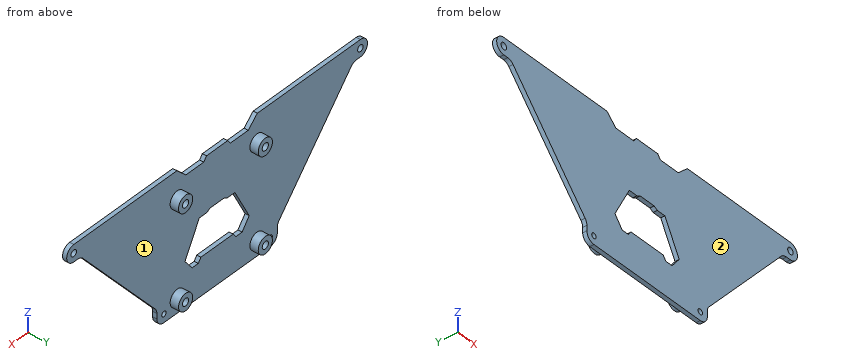
Autodesk Inventor part; units mm, degrees
ref_plane "YZ Plane" through (0, 0, 0) normal (1, 0, 0) x (0, 1, 0)
ref_plane "XZ Plane" through (0, 0, 0) normal (0, 1, 0) x (-1, 0, 0)
ref_plane "XY Plane" through (0, 0, 0) normal (0, 0, 1) x (1, 0, 0)
sketch "Sketch1" plane through (0, 0, 0) normal (0, 1, 0) x (-1, 0, 0)
  circle A0 centre (-13, 3.6355) radius 1.25
  circle A1 centre (47, 3.6355) radius 1.25
  circle A2 centre (-63.9, 60.95) radius 1.55
  circle A3 centre (-63.9, 60.95) radius 1.5
  circle A4 centre (97.9, 60.95) radius 1.55
  circle A5 centre (97.9, 60.95) radius 1.5
  arc A6 (47, -0.3645) -> (51, 3.6355) centre (47, 3.6355) ccw
  arc A7 (-17, 3.6355) -> (-13, -0.3645) centre (-13, 3.6355) ccw
  arc A8 (-63.9, 64.95) -> (-63.9, 56.95) centre (-63.9, 60.95) ccw
  arc A9 (97.9, 56.95) -> (97.9, 64.95) centre (97.9, 60.95) ccw
  line L0 (-13, -0.3645) -> (47, -0.3645)
  line L1 (-63.9, 64.95) -> (97.9, 64.95)
  line L2 (-17, 3.6355) -> (-17, 6.1391)
  line L3 (51, 3.6355) -> (51, 6.1391)
  arc A10 (51, 3.6355) -> (47, -0.3645) centre (47, 3.6355) ccw construction
  arc A11 (-13, -0.3645) -> (-17, 3.6355) centre (-13, 3.6355) ccw construction
  line L4 (-63.9, 56.95) -> (-61.722, 56.95)
  line L5 (97.9, 56.95) -> (95.722, 56.95)
  line L6 (92.7041, 55.5753) -> (51.9821, 8.7645)
  line L7 (-58.7041, 55.5753) -> (-17.9821, 8.7645)
  arc A12 (-58.7041, 55.5753) -> (-61.722, 56.95) centre (-61.722, 52.95) ccw
  arc A13 (95.722, 56.95) -> (92.7041, 55.5753) centre (95.722, 52.95) ccw
  arc A14 (51.9821, 8.7645) -> (51, 6.1391) centre (55, 6.1391) ccw
  arc A15 (-17, 6.1391) -> (-17.9821, 8.7645) centre (-21, 6.1391) ccw
  arc A16 (-63.9, 56.95) -> (-63.9, 64.95) centre (-63.9, 60.95) ccw construction
  arc A17 (97.9, 64.95) -> (97.9, 56.95) centre (97.9, 60.95) ccw construction
  point P0 (0, 0)
  point P1 (17, 90.5)
  dimension "d0" = 2.5
  dimension "d1" = 2.5
  dimension "d2" = 3
  dimension "d3" = 3
  dimension "d4" = 8
  dimension "d5" = 8
  dimension "d6" = 8
  dimension "d7" = 8
  dimension "d8" = 60
  dimension "d18" = 4
extrude "Extrusion1" add sketch "Sketch1" along normal blind 2 contours L0 A7 L2 A15 L7 A12 L4 A8 L1 A9 L5 A13 L6 A14 L3 A6
sketch "Sketch2" plane through (0, 2, 0) normal (0, 1, 0) x (1, 0, 0)
  circle A0 centre (13, -3.6355) radius 1.25
  circle A1 centre (-47, -3.6355) radius 1.25
  circle A2 centre (-39.5, -6.6355) radius 4
  circle A3 centre (5.5, -6.6355) radius 4
  circle A4 centre (5.5, -51.6355) radius 4
  circle A5 centre (-39.5, -51.6355) radius 4
  line L0 (13, 0.3645) -> (-47, 0.3645)
  circle A6 centre (-39.5, -6.6355) radius 1.75
  circle A7 centre (5.5, -6.6355) radius 1.75
  circle A8 centre (5.5, -51.6355) radius 1.75
  circle A9 centre (-39.5, -51.6355) radius 1.75
  point P0 (0, 0)
  dimension "d21" = 60
  dimension "d22" = 8
  dimension "d23" = 8
  dimension "d24" = 8
  dimension "d25" = 8
  dimension "d26" = 45
  dimension "d27" = 45
  dimension "d28" = 45
  dimension "d29" = 7
  dimension "d30" = 45
  dimension "d31" = 7.5
  dimension "d32" = 3.5
  dimension "d33" = 3.5
  dimension "d34" = 3.5
  dimension "d35" = 3.5
extrude "Extrusion2" add sketch "Sketch2" along normal blind 4 contours A2 | A3 | A4 | A5
sketch "Sketch3" plane through (0, 2, 0) normal (0, 1, 0) x (1, 0, 0)
  circle A0 centre (13, -3.6355) radius 1.55 construction
  line L0 (13, -3.6355) -> (-2, 2) construction
  line L1 (-2, 2) -> (-2, 4) construction
  line L2 (-2, 2) -> (-2, 4) construction
  line L3 (-2, 4) -> (6, 6.8723) construction
  line L4 (9.8, 6.8723) -> (53.9673, -18.6277) construction
  line L5 (6, 6.8723) -> (9.8, 6.8723) construction
  line L6 (9.8, 6.8723) -> (53.9673, -18.6277) construction
  line L7 (57.4673, -24.6899) -> (57.0036, -33.6779) construction
  line L8 (53.9673, -18.6277) -> (57.4673, -24.6899) construction
  line L9 (57.4673, -24.6899) -> (57.0036, -33.6779) construction
  line L10 (75.376, -65.5) -> (80.5, -65.5) construction
  line L11 (57.0036, -33.6779) -> (75.376, -65.5) construction
  line L12 (75.376, -65.5) -> (6.5, -65.7) construction
  line L13 (6.5, -65.7) -> (6.2893, -65.5) construction
  line L14 (0.6, -60.1) -> (-9.5, -60.1)
  line L15 (-9.5, -60.1) -> (-11, -62.1)
  line L16 (-9.5, -60.1) -> (-11, -62.1)
  line L17 (-23, -62.1) -> (-11, -62.1)
  line L18 (-11, -62.1) -> (-23, -62.1)
  line L19 (-24.5, -60.1) -> (-23, -62.1)
  line L20 (-23, -62.1) -> (-24.5, -60.1)
  line L21 (-34.6, -60.1) -> (-24.5, -60.1)
  line L22 (-24.5, -60.1) -> (-34.6, -60.1)
  line L23 (-40.5, -71.9) -> (-40.5, -65.7) construction
  line L24 (-34.6, -60.1) -> (-39.7098, -64.95)
  line L25 (-114.5, -65.5) -> (-109.376, -65.5) construction
  line L26 (-40.5, -65.7) -> (-109.376, -65.5) construction
  line L27 (-109.376, -65.5) -> (-91.0036, -33.6779) construction
  line L28 (-87.9673, -18.6277) -> (-91.4673, -24.6899) construction
  line L29 (-91.0036, -33.6779) -> (-91.4673, -24.6899) construction
  line L30 (-91.4673, -24.6899) -> (-87.9673, -18.6277) construction
  line L31 (-40, 6.8723) -> (-43.8, 6.8723) construction
  line L32 (-87.9673, -18.6277) -> (-43.8, 6.8723) construction
  line L33 (-43.8, 6.8723) -> (-40, 6.8723) construction
  line L34 (-32, 4) -> (-40, 6.8723) construction
  line L35 (-40, 6.8723) -> (-32, 4) construction
  line L36 (-32, 4) -> (-32, 2) construction
  line L37 (-32, 2) -> (-2, 2) construction
  line L38 (-6.4, -15.5) -> (-2.8831, -15.5)
  line L39 (-2.8831, -15.5) -> (-6.4, -15.5)
  line L40 (-26.1, -17.5) -> (-7.9, -17.5)
  line L41 (-6.4, -15.5) -> (-7.9, -17.5)
  line L42 (-7.9, -17.5) -> (-26.1, -17.5)
  line L43 (-31.1169, -15.5) -> (-27.6, -15.5)
  line L44 (-26.1, -17.5) -> (-27.6, -15.5)
  line L45 (-35.1306, -20.7029) -> (-31.1169, -15.5)
  line L46 (-27.6, -15.5) -> (-31.1169, -15.5)
  line L47 (-31.1169, -15.5) -> (-35.1306, -20.7029)
  line L48 (-35.1306, -20.7029) -> (-27.0449, -36)
  line L49 (-22.7189, -36) -> (-27.0449, -36)
  line L50 (-27.0449, -36) -> (-22.7189, -36)
  line L51 (-20.9689, -37) -> (-22.7189, -36)
  line L52 (-22.7189, -36) -> (-20.9689, -37)
  line L53 (-13.0311, -37) -> (-20.9689, -37)
  line L54 (-20.9689, -37) -> (-13.0311, -37)
  line L55 (-11.2811, -36) -> (-13.0311, -37)
  line L56 (-13.0311, -37) -> (-11.2811, -36)
  line L57 (-6.9551, -36) -> (-11.2811, -36)
  line L58 (-11.2811, -36) -> (-6.9551, -36)
  line L59 (1.1306, -20.7029) -> (-6.9551, -36)
  line L60 (-6.9551, -36) -> (1.1306, -20.7029)
  line L61 (1.1306, -20.7029) -> (-2.8831, -15.5)
  circle A1 centre (13, -3.6355) radius 1.25
  line L62 (-97.9, -64.95) -> (63.9, -64.95)
  line L63 (5.7098, -64.95) -> (-39.7098, -64.95)
  line L64 (5.7098, -64.95) -> (0.6, -60.1)
  point P0 (0, 0)
  point P1 (17, 90.5)
extrude "Extrusion3" cut sketch "Sketch3" against normal up to next contours L64 L62 L24 L21 L19 L17 L15 L14 | L38 L61 L59 L57 L55 L53 L51 L49 L48 L45 L43 L44 L40 L41
equation "\"d31\" = -0.5 * d26 + 0.5 * d21"
properties part number "ElectronicsMount - BoltOnStyle"
For this review, take the finished solid that the model builds, in its own axes (mm). Face numbers are marked on the shaded views. A direction names the side the tool comes from. Give positions to 0.01 mm unless a question says otherwise; leave off trailing zeros. Loops run counter-clockwise (first coordinate to the right, second up) from the corner with the lowest first, then second, coordinate; pieces in that order, holes last. Notation, with made-up numbers: (85.5, 48.5) -> (94.5, 48.5) arc R13 ccw to (94.5, 68.5) -> close; hole circle Ø7 at (41.25, 80.25). An arc over 180 degrees is marked (long way). One line per question, with ' | ' between items.
1) We need section D-D (x = 44). Write out the cut boundary in (y, z).
Resolved:
outline: (0, 38.67) -> (2, 38.67) -> (2, 64.95) -> (0, 64.95) -> close
2) For the marked faces 1 and 2, list the 3-axis set-ups (+Z, -Z, +X, -X, +Y, -Y) from which the entire face can be reached by the end or side of a thin tool; tool diameter is ignored.
Resolved:
face 1: +Y | face 2: +Z, -Z, +X, -X, -Y
3) We need section B-B (z = 22.5). Write out the cut boundary in (x, y), plus the area to 3 significant figures.
Resolved:
outline: (-63.93, 0) -> (-34.18, 0) -> (-34.18, 2) -> (-63.93, 2) -> close; (0.18, 0) -> (29.93, 0) -> (29.93, 2) -> (0.18, 2) -> close | area: 119 mm2
4) We need section C-C (x = -77.5). Write out the cut boundary in (y, z), plus the area to 3 significant figures.
Resolved:
outline: (0, 38.1) -> (2, 38.1) -> (2, 64.95) -> (0, 64.95) -> close | area: 53.7 mm2
5) Insertion check: pin 1 Ø4 at (x, z) = (0, 44.5) entering from +Y; pin 2 Ø3 at (x, y) = (1, 5) entering from -Z; pin 3 Ø1 at (x, y) = (-4, 1) entering from +Z. Each pin has a flat end and moves straight along its axis. Give the tip position at first contact, or say it passes through.
Resolved:
pin 1: stops at y = 2 | pin 2: stops at z = 3.99 | pin 3: stops at z = 60.1
6) We need section A-A (y = 3.35). Write out the cut boundary in (x, z), plus the area to 3 significant figures.
Resolved:
outline: circle Ø8 at (-39.5, 6.64); circle Ø8 at (-39.5, 51.64); circle Ø8 at (5.5, 6.64); circle Ø8 at (5.5, 51.64); hole circle Ø3.5 at (-39.5, 6.64); hole circle Ø3.5 at (-39.5, 51.64); hole circle Ø3.5 at (5.5, 6.64); hole circle Ø3.5 at (5.5, 51.64) | area: 163 mm2
7) To check wall thickness, follow probe 1 along Z at (x, y) = (-39.5, 4.2); probe 2 along X at (y, z) = (3.15, 6); probe 3 along X at (y, z) = (2.7, 5.5). State the ranges of each line that lie inside material, in increasing order.
Resolved:
probe 1: z = 2.64 to 4.89, 8.39 to 10.64, 47.64 to 49.89, 53.39 to 55.64 | probe 2: x = -43.45 to -41.13, -37.87 to -35.55, 1.55 to 3.87, 7.13 to 9.45 | probe 3: x = -43.34 to -40.83, -38.17 to -35.66, 1.66 to 4.17, 6.83 to 9.34
